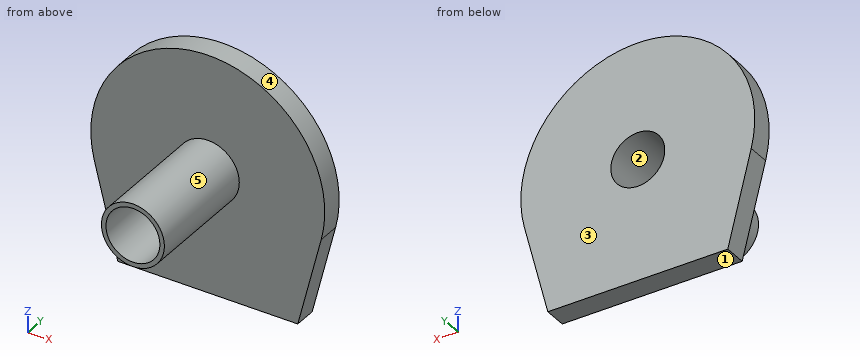
```python
from build123d import *

# Parameters (mm, degrees)
F0_R     = 3
F1_DEPTH = 2.5
F2_R     = 3.5
F2_R_2   = 3
F3_DEPTH = 13


with BuildPart() as f1:
    # F0 (on Front) → F1 (new body)
    with BuildSketch(Plane.XZ):
        with BuildLine():
            Line((10, -13.5), (12.604617, -3.181765))
            ThreePointArc((12.604617, -3.181765), (0, 13), (-12.604617, -3.181765))
            Line((-12.604617, -3.181765), (-10, -13.5))
            Line((-10, -13.5), (10, -13.5))
        make_face()
        Circle(F0_R, mode=Mode.SUBTRACT)
    extrude(amount=F1_DEPTH)

    # F2 (on face) → F3 (join)
    with BuildSketch(Plane.XZ.offset(2.5)):
        Circle(F2_R)
        Circle(F2_R_2, mode=Mode.SUBTRACT)
    extrude(amount=F3_DEPTH)


solid = f1.part
```
Can you work these out from the model? Positions are in its coordinate system, mm. Face numbers are marked on the shaded views. A direction names the side the tool comes from. Round coordinates to 2 decimals unless told otherwise and drop trailing zeros. Loops run counter-clockwise (first coordinate to the right, second up) from the corner with the lowest first, then second, coordinate; pieces in that order, holes last.
Item 1: If we mould it in two halves opening along Z, with no side actions, what happens to the marked faces 1, 2 and 3? For each: +Z half, -Z half, draft (parallel to the pull), parting line (faces both ways), or undercut.
Item 2: Suppose I cut it at A-A, the plane x = 0. Write out the boundary of the cut face in (y, z), then the cut area to 4 significant figures.
Item 3: Please list where these lines run through material, in increasing order: L1, parallel to Z at x = 0, y = -10; L2, parallel to Y at x = 9.75, z = -8; L3, parallel to Z at x = -1.5, y = -10.
Item 4: Suppose I cut it at D-D, the plane x = 9.25. Write out the boundary of the cut face in (y, z), then the cut area to 3 significant figures.
Item 5: Will these pins go through, and if not, where does the flat tip stop? pin 1 Ø4 at (x, z) = (-5.5, -1) entering from -Y; pin 2 Ø1 at (x, y) = (-2, -6) entering from +Z; pin 3 Ø2 at (y, z) = (-9, 2) entering from -X.
Item 6: Which directions (+Z, -Z, +X, -X, +Y, -Y) give clear straight access to the entire face, cutting with the end or side of a thin tool? Please do the marked faces 4 and 5.
Item 7: Suppose I cut it at B-B, the plane z = 0. Write out the boundary of the cut face in (x, y), then the cut area to 3 significant figures.
Item 8: Suppose I cut it at C-C, the plane y = -7.25. Write out the boundary of the cut face in (x, z).
Reported:
1. face 1: -Z half
1. face 2: undercut
1. face 3: draft
2. outline: (-15.5, -3.5) - (-2.5, -3.5) - (-2.5, -13.5) - (0, -13.5) - (0, -3) - (-15.5, -3) - close; (-15.5, 3) - (0, 3) - (0, 13) - (-2.5, 13) - (-2.5, 3.5) - (-15.5, 3.5) - close
2. area: 64.25 mm2
3. L1: z = -3.5 to -3, 3 to 3.5
3. L2: y = -2.5 to 0
3. L3: z = -3.16 to -2.6, 2.6 to 3.16
4. outline: (-2.5, -13.5) - (0, -13.5) - (0, 9.13) - (-2.5, 9.13) - close
4. area: 56.6 mm2
5. pin 1: stops at y = -2.5
5. pin 2: stops at z = 3.16
5. pin 3: stops at x = -3.35
6. face 4: +Y, -Y
6. face 5: -Y
7. outline: (-13, -2.5) - (-3.5, -2.5) - (-3.5, -15.5) - (-3, -15.5) - (-3, 0) - (-13, 0) - close; (3, -15.5) - (3.5, -15.5) - (3.5, -2.5) - (13, -2.5) - (13, 0) - (3, 0) - close
7. area: 63.0 mm2
8. outline: circle Ø7 at (0, 0); hole circle Ø6 at (0, 0)
